from build123d import *

# Parameters (mm, degrees)
SZKIC1_W                    = 115
SZKIC1_H                    = 50
SZKIC1_R                    = 14
DODANIE_WYCI_GNI_CIE1_DEPTH = 35
SZKIC2_R                    = 17.5
WYTNIJ_WYCI_GNI_CIE1_DEPTH  = 12
SZKIC3_R                    = 17.5
WYTNIJ_WYCI_GNI_CIE2_DEPTH  = 12
SZKIC4_R                    = 3.25
WYTNIJ_WYCI_GNI_CIE3_DEPTH  = 36
SZKIC5_W                    = 15
SZKIC5_H                    = 50
WYTNIJ_WYCI_GNI_CIE4_DEPTH  = 17.5
SFAZOWANIE1_SIZE            = 0.5


with BuildPart() as part:
    # Szkic1 → Dodanie-wyciągnięcie1 (new body)
    with BuildSketch(Plane.XY):
        Rectangle(SZKIC1_W, SZKIC1_H)
        Circle(SZKIC1_R, mode=Mode.SUBTRACT)
    extrude(amount=DODANIE_WYCI_GNI_CIE1_DEPTH)

    # Szkic2 → Wytnij-wyciągnięcie1 (cut)
    with BuildSketch(Plane.XY.offset(35)):
        Circle(SZKIC2_R)
    extrude(amount=-WYTNIJ_WYCI_GNI_CIE1_DEPTH, mode=Mode.SUBTRACT)

    # Szkic3 → Wytnij-wyciągnięcie2 (cut)
    with BuildSketch(Plane(origin=(0, 0, 0), x_dir=(-1, 0, 0), z_dir=(0, 0, -1))):
        Circle(SZKIC3_R)
    extrude(amount=-WYTNIJ_WYCI_GNI_CIE2_DEPTH, mode=Mode.SUBTRACT)

    # Szkic4 → Wytnij-wyciągnięcie3 (cut, through all)
    with BuildSketch(Plane(origin=(0, 0, 0), x_dir=(-1, 0, 0), z_dir=(0, 0, -1))):
        with Locations((-50, 15)):
            Circle(SZKIC4_R)
        with Locations((-50, -15)):
            Circle(SZKIC4_R)
        with Locations((50, 15)):
            Circle(SZKIC4_R)
        with Locations((50, -15)):
            Circle(SZKIC4_R)
    extrude(amount=-WYTNIJ_WYCI_GNI_CIE3_DEPTH, mode=Mode.SUBTRACT)

    # Szkic5 → Wytnij-wyciągnięcie4 (cut)
    with BuildSketch(Plane.XY.offset(35)):
        with Locations((50, 0)):
            Rectangle(SZKIC5_W, SZKIC5_H)
        with Locations((-50, 0)):
            Rectangle(SZKIC5_W, SZKIC5_H)
    extrude(amount=-WYTNIJ_WYCI_GNI_CIE4_DEPTH, mode=Mode.SUBTRACT)

    # Sfazowanie1
    sfazowanie1_edges = [part.edges().sort_by_distance(p)[0] for p in [
        (-17.5, 0, 35),
        (17.5, 0, 0),
    ]]
    chamfer(sfazowanie1_edges, length=SFAZOWANIE1_SIZE)


solid = part.part
CAD build for the part. Positions are in the model's coordinates, mm. A direction names the side the tool comes from. Give positions to 0.01 mm unless a question says otherwise; leave off trailing zeros. Write each loop counter-clockwise with the first axis right and the second up, starting at its lowest first coordinate (ties: lowest second). Pieces come first, ordered by that corner, then holes. Notation, with made-up numbers: (34, 88.5) - (50, 88.5) arc R19 ccw to (50, 92.5) - close; hole circle Ø10 at (-20, 40). An arc over 180 degrees is marked (long way). Put each result on its own line as item: value.
(1) Tool access for faces 5 (the flat face through (-8, 12, 23)), 6 (the flat face through (-42.5, 0, 26)), 7 (the cylindrical face through (13.887, -10.648, 6.17)), 8 (the flat face through (50, 0, 17.5)): list every direction of +Z, -Z, +X, -X, +Y, -Y with a clear straight run to the whole face (end or side of a thin tool).
Working result:
face 5: +Z
face 6: +Z, -X, +Y, -Y
face 7: -Z
face 8: +Z, +X, +Y, -Y
(2) Saw through at C-C (y = 0). List the corners of the cut face in (x, z).
Working result:
outline: (-57.5, 0) - (-18, 0) - (-17.5, 0.5) - (-17.5, 12) - (-14, 12) - (-14, 23) - (-17.5, 23) - (-17.5, 34.5) - (-18, 35) - (-42.5, 35) - (-42.5, 17.5) - (-57.5, 17.5) - close; (14, 12) - (17.5, 12) - (17.5, 0.5) - (18, 0) - (57.5, 0) - (57.5, 17.5) - (42.5, 17.5) - (42.5, 35) - (18, 35) - (17.5, 34.5) - (17.5, 23) - (14, 23) - close
(3) Drop flat-ended pins along their axis: pin 1 Ø7.5 at (x, y) = (51, -7.5) entering from +Z; pin 2 Ø19 at (y, z) = (1, 30) entering from +X; pin 3 Ø9 at (y, z) = (7.5, 25) entering from -X. Give the stop position or say it passes through.
Working result:
pin 1: z = 17.5
pin 2: x = 42.5
pin 3: x = -42.5
(4) Saw through at B-B (z = 6). List the corners of the cut face in (x, y).
Working result:
outline: (-57.5, -25) - (57.5, -25) - (57.5, 25) - (-57.5, 25) - close; hole circle Ø6.5 at (-50, -15); hole circle Ø6.5 at (-50, 15); hole circle Ø35 at (0, 0); hole circle Ø6.5 at (50, -15); hole circle Ø6.5 at (50, 15)
(5) Saw through at D-D (z = 25.5). List the corners of the cut face in (x, y).
Working result:
outline: (-42.5, -25) - (42.5, -25) - (42.5, 25) - (-42.5, 25) - close; hole circle Ø35 at (0, 0)
(6) Wall check: L1, parallel to Y at x = 50, z = 9.5; L2, parallel to Y at x = 0, z = 31.5; L3, parallel to Z at x = -9, y = -14.5. Give the ranges that are in metal, low to high.
Working result:
L1: -25 to -18.25, -11.75 to 11.75, 18.25 to 25
L2: -25 to -17.5, 17.5 to 25
L3: 12 to 23
(7) Pull direction Y, two halves, no side cores. Call faces 1 (the cylindrical face through (-13.887, -10.648, 28.83)), 2 (the flat face through (8, 12, 12)), 3 (the flat face through (-1, 25, 17)), 4 (the flat face through (-14, -16, 0)): released by +Y, released by -Y, zero draft, split by the parting line, or undercut.
Working result:
face 1: undercut
face 2: undercut
face 3: released by +Y
face 4: zero draft
(8) Saw through at A-A (x = 0). List the corners of the cut face in (y, z).
Working result:
outline: (-25, 0) - (-18, 0) - (-17.5, 0.5) - (-17.5, 12) - (-14, 12) - (-14, 23) - (-17.5, 23) - (-17.5, 34.5) - (-18, 35) - (-25, 35) - close; (14, 12) - (17.5, 12) - (17.5, 0.5) - (18, 0) - (25, 0) - (25, 35) - (18, 35) - (17.5, 34.5) - (17.5, 23) - (14, 23) - close
